For this review, take the finished solid that the model builds, in its own axes (mm). Round coordinates to 2 decimals unless told otherwise and drop trailing zeros. Order: outer loops, then holes, each group sorted by start corner. A loop starts at its lowest first (then second) coordinate and runs counter-clockwise, first axis right, second up. Notation, with made-up numbers: M 16,-10.5 L 36,-10.5 A31 cw 36,19.5 Z; hole C -38,17 d6. An arc over 180 degrees is marked long. Use a Markdown table: item, result.
from build123d import *

# Parameters (mm, degrees)
BOSS_EXTRUDE1_DEPTH = 6.35


with BuildPart() as part:
    # Sketch1 → Boss-Extrude1 (new body)
    with BuildSketch(Plane(origin=(0, 0, 0), x_dir=(1, 0, 0), z_dir=(0, 1, 0))):
        with BuildLine():
            Line((127.578922036, 62.921077964), (190.5, 0))
            Line((190.5, 0), (558.8, 0))
            Line((558.8, 0), (621.721077964, 62.921077964))
            ThreePointArc((621.721077964, 62.921077964), (639.520218393, 109.779781607), (686.378922036, 127.578922036))
            Line((686.378922036, 127.578922036), (749.3, 190.5))
            Line((749.3, 190.5), (749.3, 558.8))
            Line((749.3, 558.8), (686.378922036, 621.721077964))
            ThreePointArc((686.378922036, 621.721077964), (639.520218393, 639.520218393), (621.721077964, 686.378922036))
            Line((621.721077964, 686.378922036), (558.8, 749.3))
            Line((558.8, 749.3), (190.5, 749.3))
            Line((190.5, 749.3), (127.578922036, 686.378922036))
            ThreePointArc((127.578922036, 686.378922036), (109.779781607, 639.520218393), (62.921077964, 621.721077964))
            Line((62.921077964, 621.721077964), (0, 558.8))
            Line((0, 558.8), (0, 190.5))
            Line((0, 190.5), (62.921077964, 127.578922036))
            ThreePointArc((62.921077964, 127.578922036), (109.779781607, 109.779781607), (127.578922036, 62.921077964))
        make_face()
    extrude(amount=BOSS_EXTRUDE1_DEPTH)


solid = part.part
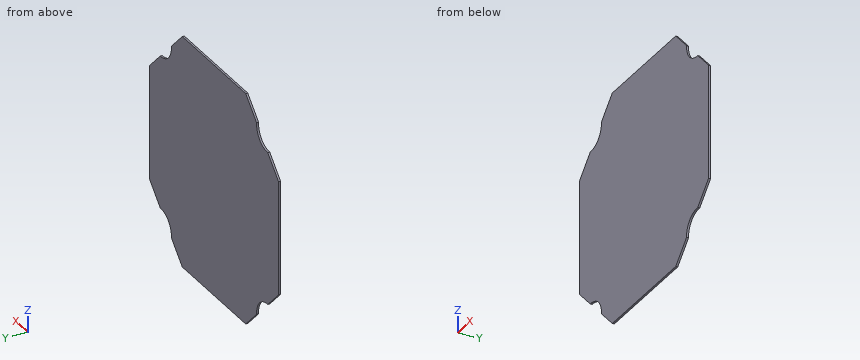
Q1. Add section B-B (x = 160). Write out the cut boundary in (y, z), then the cut area to 3 significant figures.
Determined:
| item | result |
|---|---|
| outline | M 0,-718.8 L 6.35,-718.8 L 6.35,-30.5 L 0,-30.5 Z |
| area | 4,370 mm^2 |
Q2. Add section A-A (y = 3). Write out the cut boundary in (x, z), then the cut area to 3 significant figures.
Determined:
| item | result |
|---|---|
| outline | M 0,-558.8 L 62.92,-621.72 A61.14 cw 127.58,-686.38 L 190.5,-749.3 L 558.8,-749.3 L 621.72,-686.38 A61.14 cw 686.38,-621.72 L 749.3,-558.8 L 749.3,-190.5 L 686.38,-127.58 A61.14 cw 621.72,-62.92 L 558.8,0 L 190.5,0 L 127.58,-62.92 A61.14 cw 62.92,-127.58 L 0,-190.5 Z |
| area | 484,000 mm^2 |
Q3. Add section C-C (z = -605). Write out the cut boundary in (x, y).
Determined:
| item | result |
|---|---|
| outline | M 46.2,0 L 703.1,0 L 703.1,6.35 L 46.2,6.35 Z |
Q4. Clearance check with a flat-ended pin moving along its axis: pin 1 (3 mm diameter, centred on y = 3, z = -616.5, fed in from +X). State where the tip first meets the part, or that it passes through.
Determined:
| item | result |
|---|---|
| pin 1 | stops at x = 693.1 |
Q5. Wall thickness on line 1 along X through (y, z) = (2, -72); line 2 along X through (y, z) = (6.25, -170); line 3 along Z through (x, y) = (703.5, 1.25): over which ranges is each line inside the solid? List them lowest first. Write a range as [from, to].
Determined:
| item | result |
|---|---|
| line 1 | x = [127.44, 621.86] |
| line 2 | x = [20.5, 728.8] |
| line 3 | z = [-604.6, -144.7] |
